from build123d import *

# Parameters (mm, degrees)
F0_W           = 76.2
F0_H           = 101.6
F1_DEPTH       = 3.175
F3_D           = 4.9784
F3_CSINK_D     = 9.1186
F3_CSINK_ANGLE = 82


with BuildPart() as f1:
    # F0 (on Right) → F1 (new body)
    with BuildSketch(Plane.YZ):
        Rectangle(F0_W, F0_H)
    extrude(amount=F1_DEPTH)

    # F3 (through all)
    with Locations(Plane.YZ.offset(3.175)):
        with Locations((-28.575, 41.275), (28.575, 41.275), (9.525, -41.275), (-9.525, -41.275)):
            CounterSinkHole(F3_D / 2, F3_CSINK_D / 2, counter_sink_angle=F3_CSINK_ANGLE)


solid = f1.part
CAD build for the part. Positions are in the model's coordinates, mm. Coordinates: 2 decimals unless noted, no trailing zeros. Write each loop counter-clockwise with the first axis right and the second up, starting at its lowest first coordinate (ties: lowest second). Pieces come first, ordered by that corner, then holes. Notation, with made-up numbers: M -29,9 L 9,9 A4 ccw 9,14 Z; hole C -2,-10.75 d7. An arc over 180 degrees is marked long. Answer as a JSON object with one key per item and string values. Group by question number.
1) Mould opens along Y. For faces 1 (the face through (2, 38.1, -1)), 2 (the face through (0, -1, 1)), 3 (the face through (0.391, -8.985, -43.705)), 4 (the face through (0.91, -10.92, -39.09)) say: +Y half, -Y half, draft (parallel to the pull), parting line (faces both ways), or undercut.
2) Wall check: line 1 (Z direction, x = 0.5, y = -28.5); line 2 (Y direction, x = 2.5, z = 39); line 3 (Y direction, x = 2.7, z = -37.5). Give the ranges that are in metal, low to high. Write a range as from..to.
3) Saw through at A-A (x = 2.05). Write the cut outline in (y, z) (3 decimals), plus the area to 3 significant figures.
4) Pin check, flat tips, straight feed: pin 1 Ø8 at (y, z) = (-9.525, -41.275) entering from +X; pin 2 Ø6.5 at (y, z) = (28.575, 41.275) entering from +X. Stop position of each tip, or through.
Values follow:
{
 "1": {"face 1": "+Y half", "face 2": "draft", "face 3": "undercut", "face 4": "undercut"},
 "2": {"line 1": "z = -50.8..38.79, 43.76..50.8", "line 2": "y = -38.1..-31.83, -25.32..25.32, 31.83..38.1", "line 3": "y = -38.1..-11.24, -7.81..7.81, 11.24..38.1"},
 "3": {"outline": "M -38.1,-50.8 L 38.1,-50.8 L 38.1,50.8 L -38.1,50.8 Z; hole C -28.575,41.275 d7.163; hole C -9.525,-41.275 d7.163; hole C 9.525,-41.275 d7.163; hole C 28.575,41.275 d7.163", "area": "7,580 mm2"},
 "4": {"pin 1": "stops at x = 2.53", "pin 2": "stops at x = 1.67"}
}
